Autodesk Inventor part; units mm, degrees
ref_plane "YZ Plane" through (0, 0, 0) normal (1, 0, 0) x (0, 1, 0)
ref_plane "XZ Plane" through (0, 0, 0) normal (0, 1, 0) x (-1, 0, 0)
ref_plane "XY Plane" through (0, 0, 0) normal (0, 0, 1) x (1, 0, 0)
sketch "Sketch1" plane through (0, 0, 0) normal (0, 1, 0) x (-1, 0, 0)
  line L0 (-28.575, 12.7) -> (-28.575, -12.7)
  line L1 (-28.575, -12.7) -> (28.575, -12.7)
  line L2 (28.575, -12.7) -> (28.575, 12.7)
  line L3 (28.575, 12.7) -> (-28.575, 12.7)
  line L4 (-28.575, 12.7) -> (28.575, -12.7) construction
  line L5 (-28.575, -12.7) -> (28.575, 12.7) construction
  line L6 (-25.4, 9.525) -> (-25.4, -9.525)
  line L7 (-25.4, -9.525) -> (25.4, -9.525)
  line L8 (25.4, -9.525) -> (25.4, 9.525)
  line L9 (25.4, 9.525) -> (-25.4, 9.525)
  line L10 (-25.4, 9.525) -> (25.4, -9.525) construction
  line L11 (-25.4, -9.525) -> (25.4, 9.525) construction
  point P0 (0, 0)
  dimension "d0" = 25.4
  dimension "d1" = 57.15
  dimension "d2" = 3.175
  dimension "d3" = 3.175
extrude "Extrusion1" add sketch "Sketch1" along normal blind 50.8
properties part number "spacer-1x2_250"
CAD build for the part. Positions are in the model's coordinates, mm. A direction names the side the tool comes from. Coordinates: 2 decimals unless noted, no trailing zeros. Write each loop counter-clockwise with the first axis right and the second up, starting at its lowest first coordinate (ties: lowest second). Pieces come first, ordered by that corner, then holes. Notation, with made-up numbers: M 65,43 L 81,43 A27 cw 81,65 Z; hole C 51.5,36 d5. An arc over 180 degrees is marked long. Answer as a JSON object with one key per item and string values. Group by question number.
1) Pin check, flat tip, straight feed: pin 1 Ø10 at (x, z) = (20.5, 8.5) entering from +Y. Stop position of the tip, or through.
2) Saw through at C-C (x = -13.5). Write the cut outline in (y, z) (3 decimals).
3) Tool access for faces 5 (the face through (4, 50.8, -10)), 6 (the face through (0, 25, 9.525)): list every direction of +Z, -Z, +X, -X, +Y, -Y with a clear straight run to the whole face (end or side of a thin tool).
4) Mould opens along Z. For faces 1 (the face through (4, 0, -10)), 2 (the face through (0, 25, -12.7)), 3 (the face through (0, 25, -9.525)), 4 (the face through (0, 25, 12.7)) say: +Z half, -Z half, draft (parallel to the pull), parting line (faces both ways), or undercut.
5) Wall check: line 1 (X direction, y = 30.5, z = 7.25) (3 decimals); line 2 (Z direction, x = 19, y = 9) (3 decimals). Give the ranges that are in metal, low to high. Write a range as from..to.
6) Saw through at B-B (z = 6.5). Write the cut outline in (x, y) (3 decimals), plus the area to 3 significant figures.
7) Saw through at A-A (y = 4.5). Write the cut outline in (x, z) (3 decimals), plus the area to 3 significant figures.
Values follow:
{
 "1": {"pin 1": "stops at y = 50.8"},
 "2": {"outline": "M 0,-12.7 L 50.8,-12.7 L 50.8,-9.525 L 0,-9.525 Z; M 0,9.525 L 50.8,9.525 L 50.8,12.7 L 0,12.7 Z"},
 "3": {"face 5": "+Z, -Z, +X, -X, +Y", "face 6": "+Y, -Y"},
 "4": {"face 1": "draft", "face 2": "-Z half", "face 3": "undercut", "face 4": "+Z half"},
 "5": {"line 1": "x = -28.575..-25.4, 25.4..28.575", "line 2": "z = -12.7..-9.525, 9.525..12.7"},
 "6": {"outline": "M -28.575,0 L -25.4,0 L -25.4,50.8 L -28.575,50.8 Z; M 25.4,0 L 28.575,0 L 28.575,50.8 L 25.4,50.8 Z", "area": "323 mm2"},
 "7": {"outline": "M -28.575,-12.7 L 28.575,-12.7 L 28.575,12.7 L -28.575,12.7 Z; hole M -25.4,-9.525 L 25.4,-9.525 L 25.4,9.525 L -25.4,9.525 Z", "area": "484 mm2"}
}
